from build123d import *

# Parameters (mm, degrees)
SKETCH1_R           = 6
BOSS_EXTRUDE1_DEPTH = 3
CUT_EXTRUDE2_DEPTH  = 4
CIRPATTERN1_COUNT   = 10
CUT_EXTRUDE4_DEPTH  = 4


with BuildPart() as part:
    # Sketch1 → Boss-Extrude1 (new body)
    with BuildSketch(Plane.XY):
        Circle(SKETCH1_R)
    extrude(amount=BOSS_EXTRUDE1_DEPTH)

    # Sketch2 → Cut-Extrude2 (cut, through all)
    with BuildSketch(Plane(origin=(0, 0, 0), x_dir=(-1, 0, 0), z_dir=(0, 0, -1))):
        with BuildLine():
            ThreePointArc((-1.659502931, 5.765938781), (-0.768019042, 4.919153149), (-0.540379921, 3.710861024))
            ThreePointArc((-0.540379921, 3.710861024), (0, 3.75), (0.540379921, 3.710861024))
            ThreePointArc((0.540379921, 3.710861024), (0.768019042, 4.919153149), (1.659502931, 5.765938781))
            ThreePointArc((1.659502931, 5.765938781), (0, 6), (-1.659502931, 5.765938781))
        make_face()
    cut_extrude2 = extrude(amount=-CUT_EXTRUDE2_DEPTH, mode=Mode.SUBTRACT)

    # CirPattern1: Cut-Extrude2 ×10 about axis
    cirpattern1_axis = Axis((0, 0, 0), (0, 0, 1))
    for i in range(1, CIRPATTERN1_COUNT):
        add(cut_extrude2.rotate(cirpattern1_axis, i * 360 / CIRPATTERN1_COUNT), mode=Mode.SUBTRACT)

    # Sketch4 → Cut-Extrude4 (cut, through all)
    with BuildSketch(Plane(origin=(0, 0, 0), x_dir=(-1, 0, 0), z_dir=(0, 0, -1))):
        with BuildLine():
            Line((-1.322875656, 1.5), (1.322875656, 1.5))
            ThreePointArc((1.322875656, 1.5), (0, -2), (-1.322875656, 1.5))
        make_face()
    extrude(amount=-CUT_EXTRUDE4_DEPTH, mode=Mode.SUBTRACT)


solid = part.part
Check sheet for the modelled part. Datum: model origin and axes. Units: mm. Give positions to 0.01 mm unless a question says otherwise; leave off trailing zeros. Order: outer loops, then holes, each group sorted by start corner. A loop starts at its lowest first (then second) coordinate and runs counter-clockwise, first axis right, second up. Notation, with made-up numbers: M 7.5,43 L 65.5,43 A27 cw 65.5,77 Z; hole C -32.75,82.25 d7. An arc over 180 degrees is marked long. Answer as CSV lines item,"result". Start each with the question number.
Item 1: Gauge pin test, flat ends, axial feed: P1, Ø1, axis at x = -4, y = -1, coming from the -Z side; P2, Ø1, axis at y = 1, z = 1.5, coming from the -X side. Record the tip position at first contact, or that the pin passes through.
Item 2: Cross-section at A-A on y = 0. Enter the section's corners in (x, z).
Item 3: Thickness scan on line 1 (X direction, y = 0, z = 1.95); line 2 (Y direction, x = -4, z = 0.25); line 3 (Y direction, x = 4.5, z = 0.3). Record the ranges inside material, lowest first. Write a range as [from, to].
Item 4: Cross-section at D-D on x = 3.5. Enter the section's corners in (y, z), plus the area to 3 significant figures.
Item 5: Cross-section at B-B on x = 0. Enter the section's corners in (y, z), plus the area to 3 significant figures.
Item 6: Cross-section at C-C on y = 3.5. Enter the section's corners in (x, z), plus the area to 3 significant figures.
Item 7: Mould release check, pull along X, two halves, no side actions. Record for faces 1 (the face through (0.776, 4.934, 1.479)), 2 (the face through (0, 3, 0)): +X half, -X half, draft (parallel to the pull), parting line (faces both ways), or undercut.
Established:
1,P1,"stops at z = 0"
1,P2,"stops at x = -5.64"
2,outline,"M -6,0 L -2,0 L -2,3 L -6,3 Z; M 2,0 L 6,0 L 6,3 L 2,3 Z"
3,line 1,"x = [-6, -2], [2, 6]"
3,line 2,"y = [-3.69, -1.9], [-0.75, 0.75], [1.9, 3.69]"
3,line 3,"y = [-3.72, -2.32], [-0.82, 0.82], [2.32, 3.72]"
4,outline,"M -3.52,0 L -1.69,0 L -1.69,3 L -3.52,3 Z; M -1.35,0 L 1.35,0 L 1.35,3 L -1.35,3 Z; M 1.69,0 L 3.52,0 L 3.52,3 L 1.69,3 Z"
4,area,"19.1 mm^2"
5,outline,"M -3.75,0 L -2,0 L -2,3 L -3.75,3 Z; M 1.5,0 L 3.75,0 L 3.75,3 L 1.5,3 Z"
5,area,"12.0 mm^2"
6,outline,"M -4.87,0 L -3.46,0 L -3.46,3 L -4.87,3 Z; M -1.89,0 L 1.89,0 L 1.89,3 L -1.89,3 Z; M 3.46,0 L 4.87,0 L 4.87,3 L 3.46,3 Z"
6,area,"19.9 mm^2"
7,face 1,"undercut"
7,face 2,"draft"
